Geometry: final body of the model. Coordinates: model frame, mm. Coordinates: 2 decimals unless noted, no trailing zeros. Write each loop counter-clockwise with the first axis right and the second up, starting at its lowest first coordinate (ties: lowest second). Pieces come first, ordered by that corner, then holes. Notation, with made-up numbers: (29, -2.5) - (86, -2.5) arc R11 cw to (86, 4.5) - close; hole circle Ø2 at (-36.75, 87). An arc over 180 degrees is marked (long way). Put each result on its own line as item: value.
```python
from build123d import *

# Parameters (mm, degrees)
SKETCH_1_W      = 16
SKETCH_1_H      = 40
SKETCH_1_R      = 2.5
SKETCH_1_R_2    = 5
EXTRUDE_1_DEPTH = 10
FILLET_1_R      = 3


with BuildPart() as part:
    # 草图1 → 凸台-拉伸1 (new body)
    with BuildSketch(Plane.XY):
        with Locations((0, 12.5)):
            Rectangle(SKETCH_1_W, SKETCH_1_H)
        with Locations((0, 25)):
            Circle(SKETCH_1_R, mode=Mode.SUBTRACT)
        Circle(SKETCH_1_R, mode=Mode.SUBTRACT)
        with Locations((0, 12.5)):
            Circle(SKETCH_1_R_2, mode=Mode.SUBTRACT)
    extrude(amount=EXTRUDE_1_DEPTH)

    # 圆角1
    fillet_1_edges = [part.edges().sort_by_distance(p)[0] for p in [
        (8, -7.5, 5),
        (-8, -7.5, 5),
        (-8, 32.5, 5),
        (8, 32.5, 5),
    ]]
    fillet(fillet_1_edges, radius=FILLET_1_R)


solid = part.part
```
1. Ray query, probe 1 along Y at (x, z) = (0, 2.5); probe 2 along Y at (x, z) = (1.5, 8.5); probe 3 along Y at (x, z) = (3.25, 2.5). Return the intervals inside material, ascending. Write a range as from..to.
Answer below:
probe 1: y = -7.5..-2.5, 2.5..7.5, 17.5..22.5, 27.5..32.5
probe 2: y = -7.5..-2, 2..7.73, 17.27..23, 27..32.5
probe 3: y = -7.5..8.7, 16.3..32.5
2. Section query D-D (x = -3.75). Return loops of the section in (y, z), then the cut area to 3 significant figures.
Answer below:
outline: (-7.5, 0) - (9.19, 0) - (9.19, 10) - (-7.5, 10) - close; (15.81, 0) - (32.5, 0) - (32.5, 10) - (15.81, 10) - close
area: 334 mm²
3. Pin query (flat end, axial travel): pin 1 Ø5 at (x, z) = (6, 8) entering from -Y. Return the tip coordinate at first contact, or that it passes through.
Answer below:
pin 1: stops at y = -7.5
4. Section query C-C (x = 0). Return loops of the section in (y, z).
Answer below:
outline: (-7.5, 0) - (-2.5, 0) - (-2.5, 10) - (-7.5, 10) - close; (2.5, 0) - (7.5, 0) - (7.5, 10) - (2.5, 10) - close; (17.5, 0) - (22.5, 0) - (22.5, 10) - (17.5, 10) - close; (27.5, 0) - (32.5, 0) - (32.5, 10) - (27.5, 10) - close
5. Mould query, pull axis Y, two halves, no side actions, for faces 1 (the flat face through (0, -7.5, 5)), 2 (the cylindrical face through (-0.651, 17.457, 4.93)), 3 (the flat face through (0, 32.5, 5)), 4 (the cylindrical face through (-0.33, 27.48, 4.93)). Classes: +Y half, -Y half, draft (parallel to the pull), parting line (faces both ways), or undercut.
Answer below:
face 1: -Y half
face 2: undercut
face 3: +Y half
face 4: undercut
6. Section query A-A (y = -2). Return loops of the section in (x, z).
Answer below:
outline: (-8, 0) - (-1.5, 0) - (-1.5, 10) - (-8, 10) - close; (1.5, 0) - (8, 0) - (8, 10) - (1.5, 10) - close
7. Section query B-B (z = 4). Return loops of the section in (x, y).
Answer below:
outline: (-8, -4.5) arc R3 ccw to (-5, -7.5) - (5, -7.5) arc R3 ccw to (8, -4.5) - (8, 29.5) arc R3 ccw to (5, 32.5) - (-5, 32.5) arc R3 ccw to (-8, 29.5) - close; hole circle Ø10 at (0, 12.5); hole circle Ø5 at (0, 0); hole circle Ø5 at (0, 25)
